For this review, use the dimensioned drawing (mm, ordinates from the lowest corner) and the shaded views. A direction names the side the tool comes from. Round coordinates to 2 decimals unless told otherwise and drop trailing zeros. Write each loop counter-clockwise with the first axis right and the second up, starting at its lowest first coordinate (ties: lowest second). Pieces come first, ordered by that corner, then holes. Notation, with made-up numbers: (54.5, 63.5) -> (103.5, 63.5) arc R18 ccw to (103.5, 76.5) -> close; hole circle Ø10 at (29.25, 74.5). An arc over 180 degrees is marked (long way). Write each question's results on one line, items separated by ' | '. Start each with the question number.
Item 1: Tool access review of the marked faces 1 and 2: name each direction out of +Z, -Z, +X, -X, +Y, -Y from which nothing blocks a thin tool from reaching the whole face with its end or side.
Item 2: The part is to be moulded in two halves that separate along X. For the marked faces 3, 4, 5 and 6, say which applies: +X half, -X half, draft (parallel to the pull), parting line (faces both ways), or undercut.
Item 3: Add section D-D (y = 1.75). State the section outline as (x, z) points, plus the area to 3 significant figures.
Item 4: Clearance check with flat-ended pins moving along their axes: pin 1 (12 mm diameter, centred on y = 17.5, z = 58.5, fed in from -X); pin 2 (8 mm diameter, centred on x = 75, y = 15, fed in from -Z); pin 3 (2 mm diameter, centred on y = 2.5, z = 31, fed in from -X). State where each tip first meets the part, or that it passes through.
Item 5: Add section C-C (z = 50). State the section outline as (x, y) points.
Item 6: Add section A-A (x = 50). State the section outline as (y, z) points.
Item 7: To check wall thickness, follow line 1 along Z through (x, y) = (26.5, 10.25) (1 decimal); line 2 along Z through (x, y) = (66, 11.5) (1 decimal); line 3 along Y through (x, z) = (78.5, 70). State the ranges of each line that lie inside material, in increasing order.
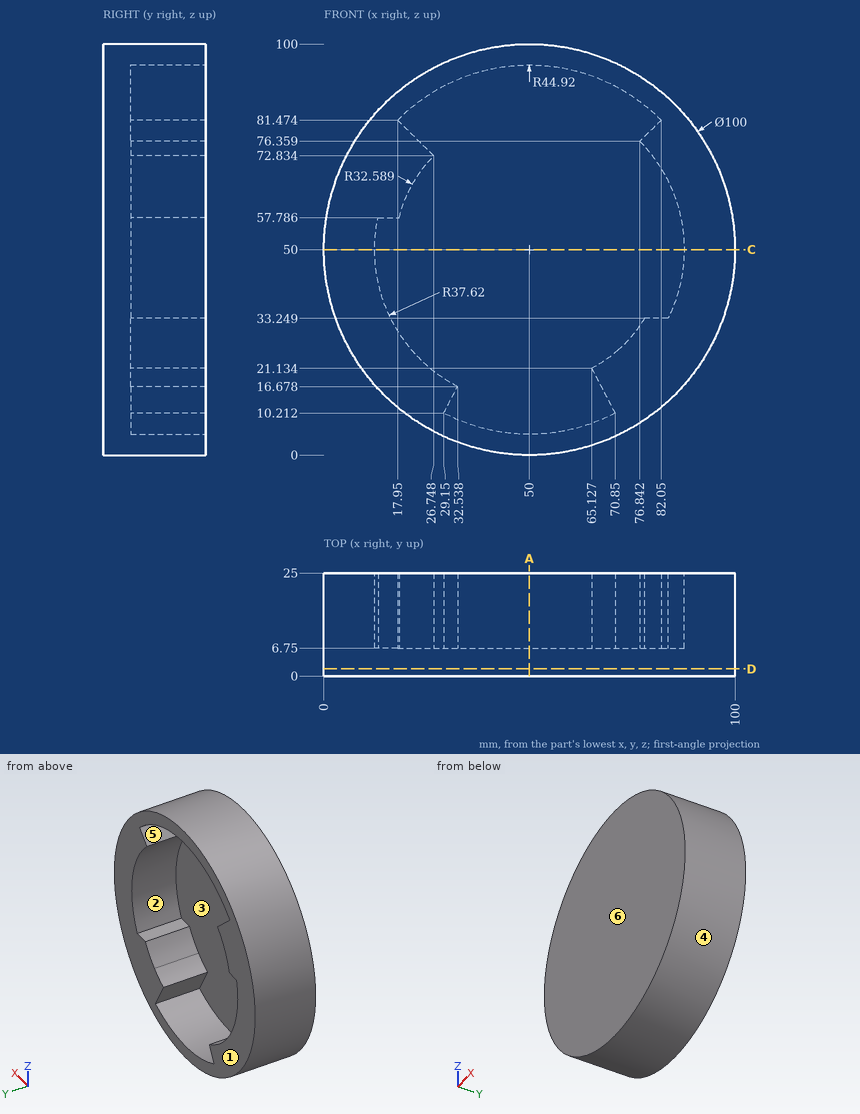
Responses:
1) face 1: +Z, -Z, +X, -X, +Y | face 2: +Y
2) face 3: undercut | face 4: parting line | face 5: undercut | face 6: draft
3) outline: circle Ø100 at (50, 50) | area: 7,850 mm^2
4) pin 1: stops at x = 0.06 | pin 2: stops at z = 4.62 | pin 3: stops at x = 3.35
5) outline: (0, 0) -> (100, 0) -> (100, 25) -> (87.62, 25) -> (87.62, 6.75) -> (12.38, 6.75) -> (12.38, 25) -> (0, 25) -> close
6) outline: (0, 0) -> (25, 0) -> (25, 5.08) -> (6.75, 5.08) -> (6.75, 94.92) -> (25, 94.92) -> (25, 100) -> (0, 100) -> close
7) line 1: z = 5.9 to 20.6, 72.6 to 73.1, 88.3 to 94.1 | line 2: z = 2.6 to 8, 19.5 to 21.6, 92 to 97.4 | line 3: y = 0 to 6.75
